```python
from build123d import *

# Parameters (mm, degrees)
SKETCH033_W     = 20
SKETCH033_H     = 20
PAD015_DEPTH    = 10
SKETCH034_R     = 2.5
HOLE009_DEPTH   = 25
SKETCH035_R     = 2.5
HOLE010_DEPTH   = 25
SKETCH036_R     = 2.5
HOLE011_DEPTH   = 25
SKETCH037_W     = 14
SKETCH037_H     = 14
POCKET009_DEPTH = 17
SKETCH038_W     = 14
SKETCH038_H     = 14
POCKET010_DEPTH = 17
SKETCH039_W     = 14
SKETCH039_H     = 14
POCKET011_DEPTH = 17


with BuildPart() as part:
    # Sketch033 → Pad015 (new body, symmetric)
    with BuildSketch(Plane.XZ):
        Rectangle(SKETCH033_W, SKETCH033_H)
    extrude(amount=PAD015_DEPTH, both=True)

    # Sketch034 (on Face1 of Pad015) → Hole009 (cut)
    with BuildSketch(Plane(origin=(0, 0, 10), x_dir=(-1, 0, 0), z_dir=(0, 0, 1))):
        Circle(SKETCH034_R)
    extrude(amount=-HOLE009_DEPTH, mode=Mode.SUBTRACT)

    # Sketch035 (on Face2 of Hole009) → Hole010 (cut)
    with BuildSketch(Plane(origin=(10, 0, 0), x_dir=(0, 0, 1), z_dir=(1, 0, 0))):
        Circle(SKETCH035_R)
    extrude(amount=-HOLE010_DEPTH, mode=Mode.SUBTRACT)

    # Sketch036 (on Face3 of Hole009) → Hole011 (cut)
    with BuildSketch(Plane(origin=(0, 10, 0), x_dir=(1, 0, 0), z_dir=(0, 1, 0))):
        Circle(SKETCH036_R)
    extrude(amount=-HOLE011_DEPTH, mode=Mode.SUBTRACT)

    # Sketch037 (on Face2 of Hole011) → Pocket009 (cut)
    with BuildSketch(Plane(origin=(10, 0, 0), x_dir=(0, 0, 1), z_dir=(1, 0, 0))):
        Rectangle(SKETCH037_W, SKETCH037_H)
    extrude(amount=-POCKET009_DEPTH, mode=Mode.SUBTRACT)

    # Sketch038 (on Face3 of Pocket009) → Pocket010 (cut)
    with BuildSketch(Plane(origin=(0, 10, 0), x_dir=(1, 0, 0), z_dir=(0, 1, 0))):
        Rectangle(SKETCH038_W, SKETCH038_H)
    extrude(amount=-POCKET010_DEPTH, mode=Mode.SUBTRACT)

    # Sketch039 (on Face1 of Pocket010) → Pocket011 (cut)
    with BuildSketch(Plane(origin=(0, 0, 10), x_dir=(-1, 0, 0), z_dir=(0, 0, 1))):
        Rectangle(SKETCH039_W, SKETCH039_H)
    extrude(amount=-POCKET011_DEPTH, mode=Mode.SUBTRACT)


solid = part.part
```
Verification items for the finished model (mm, model axes). A direction names the side the tool comes from. Give positions to 0.01 mm unless a question says otherwise; leave off trailing zeros. Loops run counter-clockwise (first coordinate to the right, second up) from the corner with the lowest first, then second, coordinate; pieces in that order, holes last.
1. Thickness scan on line 1 (Z direction, x = 8, y = -3.25); line 2 (Y direction, x = -8.85, z = 0). Record the ranges inside material, lowest first.
2. Mould release check, pull along Z, two halves, no side actions. Record for faces 4 (the flat face through (7, 0, 9)), 5 (the cylindrical face through (-8.48, 2.44, -0.54)), 6 (the flat face through (-9, 0, 10)): released by +Z, released by -Z, zero draft, split by the parting line, or undercut.
3. Set-up check for faces 1 (the flat face through (0, 9, 7)), 2 (the flat face through (-7, 2, 4)), 3 (the flat face through (0, 7, 9)): record each of +Z, -Z, +X, -X, +Y, -Y from which the full face is reachable in a straight line by a thin tool's end or side.
4. Section check B-B, the plane y = 3.5. Enter the section's corners in (x, z).
5. Go/stop test with flat-tipped pins: pin 1 Ø10 at (x, z) = (-1, 1.5) entering from +Y; pin 2 Ø3 at (x, y) = (0, 0) entering from -Z; pin 3 Ø6.5 at (y, z) = (0, 0) entering from +X. Record where each tip stops, or that it passes through.
6. Section check A-A, the plane z = 0. Enter the section's corners in (x, y), then the cut area to 3 significant figures.
Geometry says:
1. line 1: z = -10 to -7, 7 to 10
1. line 2: y = -10 to -2.5, 2.5 to 10
2. face 4: zero draft
2. face 5: undercut
2. face 6: released by +Z
3. face 1: +Y
3. face 2: none
3. face 3: +Z
4. outline: (-10, -10) - (10, -10) - (10, -7) - (-7, -7) - (-7, 10) - (-10, 10) - close; (7, 7) - (10, 7) - (10, 10) - (7, 10) - close
5. pin 1: stops at y = -7
5. pin 2: passes through
5. pin 3: stops at x = -7
6. outline: (-10, -10) - (-2.5, -10) - (-2.5, -7) - (-7, -7) - (-7, -2.5) - (-10, -2.5) - close; (-10, 2.5) - (-7, 2.5) - (-7, 10) - (-10, 10) - close; (2.5, -10) - (10, -10) - (10, -7) - (2.5, -7) - close; (7, 7) - (10, 7) - (10, 10) - (7, 10) - close
6. area: 90.0 mm2
